Print and shaded views of the part. All mm, measured from the part's lowest x, y and z. A direction names the side the tool comes from. Round coordinates to 2 decimals unless told otherwise and drop trailing zeros. Loops run counter-clockwise (first coordinate to the right, second up) from the corner with the lowest first, then second, coordinate; pieces in that order, holes last. Notation, with made-up numbers: (42, -5.75) -> (101, -5.75) arc R12 ccw to (101, 15.25) -> close; hole circle Ø4 at (-16.75, -28). An arc over 180 degrees is marked (long way). Answer as CSV lines item,"result".
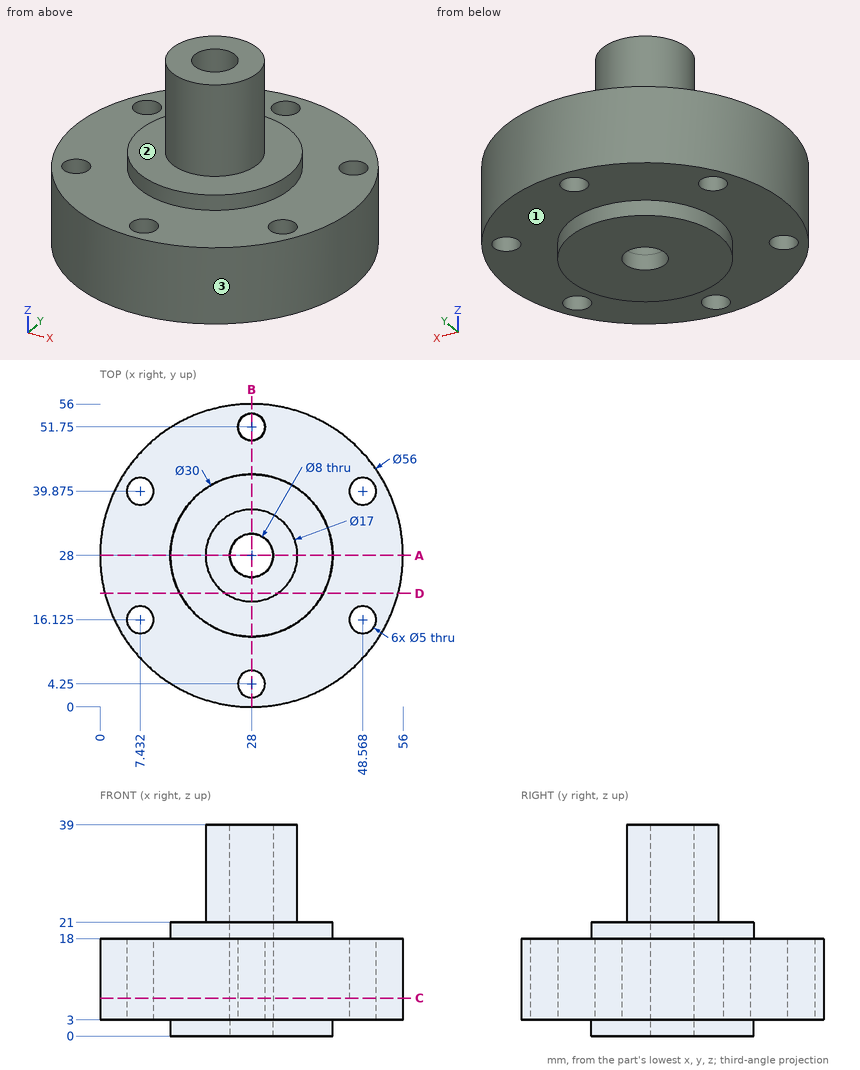
Q1. Saw through at B-B, the plane x = 28. Write the cut outline in (y, z), then the cut area to 3 significant figures.
Geometry results:
outline,"(0, 3) -> (1.75, 3) -> (1.75, 18) -> (0, 18) -> close; (6.75, 3) -> (13, 3) -> (13, 0) -> (24, 0) -> (24, 39) -> (19.5, 39) -> (19.5, 21) -> (13, 21) -> (13, 18) -> (6.75, 18) -> close; (32, 0) -> (43, 0) -> (43, 3) -> (49.25, 3) -> (49.25, 18) -> (43, 18) -> (43, 21) -> (36.5, 21) -> (36.5, 39) -> (32, 39) -> close; (54.25, 3) -> (56, 3) -> (56, 18) -> (54.25, 18) -> close"
area,"864 mm2"
Q2. Drill centre lines: line 1 along Z through (x, y) = (44.5, 40); line 2 along X through (y, z) = (15, 4.5); line 3 along X through (y, z) = (53.5, 13.5) (1 decimal). Where is each one in solid material? Low to high.
Geometry results:
line 1,"3 to 18"
line 2,"3.2 to 5.2, 9.66 to 46.34, 50.8 to 52.8"
line 3,"16.4 to 26.2, 29.8 to 39.6"
Q3. Saw through at C-C, the plane z = 7. Write the cut outline in (x, y) (3 decimals), then the cut area to 3 significant figures.
Geometry results:
outline,"circle Ø56 at (28, 28); hole circle Ø5 at (7.432, 16.125); hole circle Ø5 at (7.432, 39.875); hole circle Ø8 at (28, 28); hole circle Ø5 at (28, 4.25); hole circle Ø5 at (28, 51.75); hole circle Ø5 at (48.568, 16.125); hole circle Ø5 at (48.568, 39.875)"
area,"2,290 mm2"
Q4. Drop flat-ended pins along their axis: P1, Ø4.5, axis at x = 7.43, y = 16.12, coming from the -Z side; P2, Ø5, axis at y = 39.5, z = 12.5, coming from the -X side; P3, Ø4, axis at x = 36.5, z = 28, coming from the +Y side; P4, Ø12, axis at x = 8.5, z = 19.5, coming from the -Y side (1 decimal). Give the stop position or say it passes through.
Geometry results:
P1,"through"
P2,"x = 1.49"
P3,"y = 33.48"
P4,"y = 3.6"
Q5. Saw through at D-D, the plane y = 21. Write the cut outline in (x, z), then the cut area to 3 significant figures.
Geometry results:
outline,"(0.89, 3) -> (14.73, 3) -> (14.73, 0) -> (41.27, 0) -> (41.27, 3) -> (55.11, 3) -> (55.11, 18) -> (41.27, 18) -> (41.27, 21) -> (32.82, 21) -> (32.82, 39) -> (23.18, 39) -> (23.18, 21) -> (14.73, 21) -> (14.73, 18) -> (0.89, 18) -> close"
area,"1,150 mm2"
Q6. Which spindle directions (+Z, -Z, +X, -X, +Y, -Y) get a long thin tool onto all of the face, cutting with end or side? Do the marked faces 1, 2 and 3. Say none if no direction does.
Geometry results:
face 1,"-Z"
face 2,"+Z"
face 3,"+Z, -Z"
Q7. Saw through at A-A, the plane y = 28. Write the cut outline in (x, z).
Geometry results:
outline,"(0, 3) -> (13, 3) -> (13, 0) -> (24, 0) -> (24, 39) -> (19.5, 39) -> (19.5, 21) -> (13, 21) -> (13, 18) -> (0, 18) -> close; (32, 0) -> (43, 0) -> (43, 3) -> (56, 3) -> (56, 18) -> (43, 18) -> (43, 21) -> (36.5, 21) -> (36.5, 39) -> (32, 39) -> close"
